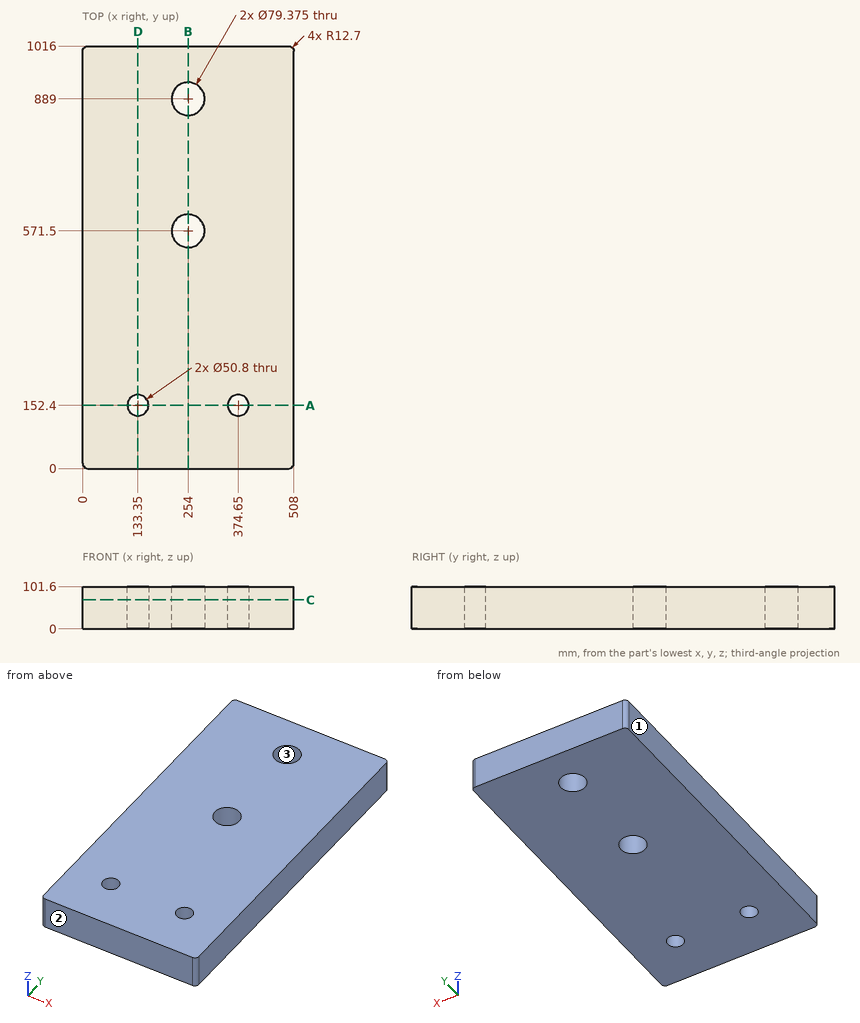
Input: dimensioned drawing with shaded views. Units: mm. Origin: part minimum x, y, z. Give positions to 0.01 mm unless a question says otherwise; leave off trailing zeros. Write each loop counter-clockwise with the first axis right and the second up, starting at its lowest first coordinate (ties: lowest second). Pieces come first, ordered by that corner, then holes. Notation, with made-up numbers: (-21, 82.25) - (20, 82.25) arc R26 ccw to (20, 98.25) - close; hole circle Ø2 at (-6, 11). An arc over 180 degrees is marked (long way). Write item = value, one per line. Start each with the question number.
1) Pin query (flat end, axial travel): pin 1 (10 mm diameter, centred on y = 214, z = 49, fed in from -X). Return the tip coordinate at first contact, or that it passes through.
2) Material intervals for L1, parallel to Y at x = 254, z = 64.5; L2, parallel to X at y = 152, z = 63; L3, parallel to X at y = 149, z = 44.5, sorted ascending. Write a range as [from, to].
3) Draft query along X for the marked faces 1, 2 and 3. Return one class per face: pulls with the +X half, pulls with the -X half, needs draft (parallel to the pull), parting line crosses it, or undercut.
4) Cut plane D-D (x = 133.35). Return loops of the section in (y, z), and give its area (3 significant figures).
5) Cut plane A-A (y = 152.4). Return loops of the section in (x, z).
6) Cut plane C-C (z = 70). Give the number of separate pieces and of enclosed holes in the cut face, and give its area (3 significant figures).
7) Cut plane B-B (x = 254). Return loops of the section in (y, z), and give its area (3 significant figures).
Answers follow:
q1.pin_1 = 0
q2.L1 = [0, 531.81], [611.19, 849.31], [928.69, 1016]
q2.L2 = [0, 107.95], [158.75, 349.25], [400.05, 508]
q2.L3 = [0, 108.18], [158.52, 349.48], [399.82, 508]
q3.face_1 = pulls with the -X half
q3.face_2 = needs draft
q3.face_3 = undercut
q4.outline = (0, 0) - (127, 0) - (127, 101.6) - (0, 101.6) - close; (177.8, 0) - (1016, 0) - (1016, 101.6) - (177.8, 101.6) - close
q4.area = 98,100 mm^2
q5.outline = (0, 0) - (107.95, 0) - (107.95, 101.6) - (0, 101.6) - close; (158.75, 0) - (349.25, 0) - (349.25, 101.6) - (158.75, 101.6) - close; (400.05, 0) - (508, 0) - (508, 101.6) - (400.05, 101.6) - close
q6.separate_pieces = 1
q6.enclosed_holes = 4
q6.area = 502,000 mm^2
q7.outline = (0, 0) - (531.81, 0) - (531.81, 101.6) - (0, 101.6) - close; (611.19, 0) - (849.31, 0) - (849.31, 101.6) - (611.19, 101.6) - close; (928.69, 0) - (1016, 0) - (1016, 101.6) - (928.69, 101.6) - close
q7.area = 87,100 mm^2
